Verification items for the finished model (mm, model axes). A direction names the side the tool comes from. Coordinates: 2 decimals unless noted, no trailing zeros. Write each loop counter-clockwise with the first axis right and the second up, starting at its lowest first coordinate (ties: lowest second). Pieces come first, ordered by that corner, then holes. Notation, with made-up numbers: (85.25, 12.5) -> (143.25, 12.5) arc R15 cw to (143.25, 26.5) -> close; hole circle Ø3 at (46.25, -4). An arc over 180 degrees is marked (long way). Write each question's results on one line, items separated by ' | '. Start each with the question number.
from build123d import *

# Parameters (mm, degrees)
SKETCH1_W           = 20
SKETCH1_H           = 20
BOSS_EXTRUDE1_DEPTH = 10
SKETCH3_W           = 19
SKETCH3_H           = 19
CUT_EXTRUDE1_DEPTH  = 20
FILLET1_R           = 0.5
SKETCH4_R           = 2
CUT_EXTRUDE2_DEPTH  = 2
SKETCH5_R           = 2
CUT_EXTRUDE3_DEPTH  = 2


with BuildPart() as part:
    # Sketch1 → Boss-Extrude1 (new body, symmetric)
    with BuildSketch(Plane(origin=(0, 0, 0), x_dir=(0, 0, -1), z_dir=(1, 0, 0))):
        with Locations((-10, 10)):
            Rectangle(SKETCH1_W, SKETCH1_H)
    extrude(amount=BOSS_EXTRUDE1_DEPTH, both=True)

    # Sketch3 → Cut-Extrude1 (cut)
    with BuildSketch(Plane(origin=(10, 0, 0), x_dir=(0, 0, -1), z_dir=(1, 0, 0))):
        with Locations((-10.5, 10.5)):
            Rectangle(SKETCH3_W, SKETCH3_H)
    extrude(amount=-CUT_EXTRUDE1_DEPTH, mode=Mode.SUBTRACT)

    # Fillet1
    fillet1_edges = [part.edges().sort_by_distance(p)[0] for p in [
        (0, 0, 0),
    ]]
    fillet(fillet1_edges, radius=FILLET1_R)

    # Sketch4 → Cut-Extrude2 (cut)
    with BuildSketch(Plane(origin=(0, 0, 0), x_dir=(-1, 0, 0), z_dir=(0, 0, -1))):
        with Locations((0, 10)):
            Circle(SKETCH4_R)
    extrude(amount=-CUT_EXTRUDE2_DEPTH, mode=Mode.SUBTRACT)

    # Sketch5 → Cut-Extrude3 (cut)
    with BuildSketch(Plane.XZ):
        with Locations((0, 10)):
            Circle(SKETCH5_R)
    extrude(amount=-CUT_EXTRUDE3_DEPTH, mode=Mode.SUBTRACT)


solid = part.part
1. Sectioned sample at D-D on x = -7.5. Record the cut outline in (y, z).
2. Sectioned sample at A-A on y = 10. Record the cut outline in (x, z), plus the area to 3 significant figures.
3. Material ranges on probe 1 along Z at (x, y) = (0, 0.5); probe 2 along Y at (x, z) = (-7.25, 16.5), recorded low to high. Write a range as from..to.
4. Depth check by flat-ended pin: pin 1 Ø3 at (x, z) = (-3, 12.5) entering from +Y; pin 2 Ø1 at (x, y) = (6.5, 12.5) entering from +Z. Enter the tip coordinate at first touch or a pass-through.
5. Tool access check on faces 1 (the flat face through (0.1, 12.5, 1)), 2 (the flat face through (0.1, 0.5, 20)). Record the directions out of +Z, -Z, +X, -X, +Y, -Y that give a thin tool (end or side, any length) a straight path to the whole face; none if there is none.
6. Sectioned sample at B-B on x = 0. Record the cut outline in (y, z).
7. Mould release check, pull along Y, two halves, no side actions. Record for faces 3 (the flat face through (10, 0.4, 5.6)), 4 (the flat face through (0, 1, 13)), 5 (the cylindrical face through (0.26, 11.983, 0.493)), 6 (the flat face through (0, 0, 13)): +Y half, -Y half, draft (parallel to the pull), parting line (faces both ways), or undercut.
Computed values:
1) outline: (0, 0.5) arc R0.5 ccw to (0.5, 0) -> (20, 0) -> (20, 1) -> (1, 1) -> (1, 20) -> (0, 20) -> close
2) outline: (-10, 0) -> (-2, 0) -> (-2, 1) -> (-10, 1) -> close; (2, 0) -> (10, 0) -> (10, 1) -> (2, 1) -> close | area: 16.0 mm^2
3) probe 1: z = 0..8, 12..20 | probe 2: y = 0..1
4) pin 1: stops at y = 1 | pin 2: stops at z = 1
5) face 1: +Z, +X, -X, +Y | face 2: +Z, +X, -X, +Y, -Y
6) outline: (0, 0.5) arc R0.5 ccw to (0.5, 0) -> (8, 0) -> (8, 1) -> (1, 1) -> (1, 8) -> (0, 8) -> close; (0, 12) -> (1, 12) -> (1, 20) -> (0, 20) -> close; (12, 0) -> (20, 0) -> (20, 1) -> (12, 1) -> close
7) face 3: draft | face 4: +Y half | face 5: undercut | face 6: -Y half
